CAD build for the part. Positions are in the model's coordinates, mm. A direction names the side the tool comes from. Coordinates: 2 decimals unless noted, no trailing zeros. Loops run counter-clockwise (first coordinate to the right, second up) from the corner with the lowest first, then second, coordinate; pieces in that order, holes last. Notation, with made-up numbers: (20, -23) -> (27, -23) arc R32 cw to (27, 5) -> close; hole circle Ø10 at (8.5, 51.5). An arc over 180 degrees is marked (long way). Write each question's results on one line, items separated by ' | '.
```python
from build123d import *

# Parameters (mm, degrees)
BOSS_EXTRUDE1_DEPTH = 12.5
SKETCH2_R           = 9.5
CUT_EXTRUDE1_DEPTH  = 24.5
CUT_EXTRUDE2_REACH  = 79.945
SKETCH3_R           = 7
CUT_EXTRUDE3_REACH  = 97.897
SKETCH4_R           = 2


with BuildPart() as part:
    # Sketch1 → Boss-Extrude1 (new, symmetric)
    with BuildSketch(Plane(origin=(0, 0, 0), x_dir=(0, 0, -1), z_dir=(1, 0, 0))):
        Polygon((0, 0), (0, -33), (-20, -33), (-20, -31), (-86.5, -31), (-86.5, -25), (-41.5, -25), (-41.5, -6), (-86.5, -6), (-86.5, 0), align=None)
    extrude(amount=BOSS_EXTRUDE1_DEPTH, both=True)

    # Sketch2 → Cut-Extrude1 (cut)
    with BuildSketch(Plane.XY.offset(41.5)):
        with Locations((0, -15.5)):
            Circle(SKETCH2_R)
    extrude(amount=-CUT_EXTRUDE1_DEPTH, mode=Mode.SUBTRACT)

    # Sketch3 → Cut-Extrude2 (cut, up to next)
    with BuildSketch(Plane.XY.offset(17), mode=Mode.PRIVATE) as cut_extrude2_sk1:
        with Locations((0, -15.5)):
            Circle(SKETCH3_R)
    cut_extrude2_tool1 = extrude(cut_extrude2_sk1.sketch, amount=-CUT_EXTRUDE2_REACH, mode=Mode.PRIVATE) & part.part
    add(cut_extrude2_tool1.solids().sort_by_distance((0, -15.5, 17))[0], mode=Mode.SUBTRACT)

    # Sketch4 → Cut-Extrude3 (cut, up to next)
    with BuildSketch(Plane(origin=(12.5, 0, 0), x_dir=(0, 0, -1), z_dir=(1, 0, 0)), mode=Mode.PRIVATE) as cut_extrude3_sk1:
        with Locations((-15, -29)):
            Circle(SKETCH4_R)
    cut_extrude3_tool1 = extrude(cut_extrude3_sk1.sketch, amount=-CUT_EXTRUDE3_REACH, mode=Mode.PRIVATE) & part.part
    # Sketch4 → Cut-Extrude3 (cut, up to next)
    with BuildSketch(Plane(origin=(12.5, 0, 0), x_dir=(0, 0, -1), z_dir=(1, 0, 0)), mode=Mode.PRIVATE) as cut_extrude3_sk2:
        with Locations((-5, -29)):
            Circle(SKETCH4_R)
    cut_extrude3_tool2 = extrude(cut_extrude3_sk2.sketch, amount=-CUT_EXTRUDE3_REACH, mode=Mode.PRIVATE) & part.part
    add(cut_extrude3_tool1.solids().sort_by_distance((12.5, -29, 15))[0], mode=Mode.SUBTRACT)
    add(cut_extrude3_tool2.solids().sort_by_distance((12.5, -29, 5))[0], mode=Mode.SUBTRACT)


solid = part.part
```
Q1. Which spindle directions (+Z, -Z, +X, -X, +Y, -Y) get a long thin tool onto all of the face, cutting with end or side? Do faces 1 (the flat face through (0, -32, 20)), 2 (the flat face through (11, -16, 41.5)), 3 (the cylindrical face through (4.38, -23.93, 29.42)), 4 (the flat face through (-12.5, -16, 33)). Say none if no direction does.
Results are:
face 1: +Z, +X, -X, -Y | face 2: +Z, +X, -X | face 3: +Z | face 4: +Z, -Z, -X, +Y, -Y
Q2. Cut at D-D on x = -3. Write the cut outline in (y, z), and give its area (3 significant figures).
Results are:
outline: (-33, 0) -> (-21.82, 0) -> (-21.82, 17) -> (-24.51, 17) -> (-24.51, 41.5) -> (-25, 41.5) -> (-25, 86.5) -> (-31, 86.5) -> (-31, 20) -> (-33, 20) -> close; (-9.18, 0) -> (0, 0) -> (0, 86.5) -> (-6, 86.5) -> (-6, 41.5) -> (-6.49, 41.5) -> (-6.49, 17) -> (-9.18, 17) -> close; hole circle Ø4 at (-29, 5); hole circle Ø4 at (-29, 15) | area: 1,180 mm^2
Q3. Drop flat-ended pins along their axis: pin 1 (1.6 mm diameter, centred on x = 1, y = -32, fed in from +Z); pin 2 (1.5 mm diameter, centred on x = 6.5, z = 40.5, fed in from +Y); pin 3 (12 mm diameter, centred on x = 8, z = 40, fed in from -Y); pin 4 (15 mm diameter, centred on x = -0.5, y = -17, fed in from +Z). Give the stop position or say it passes through.
Results are:
pin 1: z = 20 | pin 2: y = 0 | pin 3: y = -31 | pin 4: z = 17
Q4. Pull direction Z, two halves, no side cores. Call faces 5 (the flat face through (0, 0, 44)), 6 (the flat face through (0, -28, 86.5)), 7 (the cylindrical face through (0, -31, 15)): +Z half, -Z half, draft (parallel to the pull), parting line (faces both ways), or undercut.
Results are:
face 5: draft | face 6: +Z half | face 7: undercut
Q5. Cut at B-B on y = -29. Write the cut outline in (x, z).
Results are:
outline: (-12.5, 0) -> (12.5, 0) -> (12.5, 3) -> (-12.5, 3) -> close; (-12.5, 7) -> (12.5, 7) -> (12.5, 13) -> (-12.5, 13) -> close; (-12.5, 17) -> (12.5, 17) -> (12.5, 86.5) -> (-12.5, 86.5) -> close
Q6. Cut at A-A on z = 5. Write the cut outline in (x, y).
Results are:
outline: (-12.5, -33) -> (12.5, -33) -> (12.5, -31) -> (-12.5, -31) -> close; (-12.5, -27) -> (12.5, -27) -> (12.5, 0) -> (-12.5, 0) -> close; hole circle Ø14 at (0, -15.5)
Q7. Cut at C-C on z = 65. Write the cut outline in (x, y), and give its area (3 significant figures).
Results are:
outline: (-12.5, -31) -> (12.5, -31) -> (12.5, -25) -> (-12.5, -25) -> close; (-12.5, -6) -> (12.5, -6) -> (12.5, 0) -> (-12.5, 0) -> close | area: 300 mm^2
Q8. Wall check: L1, parallel to Y at x = 0, z = 29.75; L2, parallel to Y at x = 2.5, z = 5; L3, parallel to Y at x = 0, z = 12.75. Give the ranges that are in metal, low to high. Write a range as from..to.
Results are:
L1: -31..-25, -6..0 | L2: -33..-31, -27..-22.04, -8.96..0 | L3: -33..-22.5, -8.5..0
